from build123d import *

# Parameters (mm, degrees)
F1_DEPTH = 8.45


with BuildPart() as f1:
    # F0 (on Top) → F1 (new body)
    with BuildSketch(Plane.XY):
        with BuildLine():
            Line((-4.005518, -15.555335), (-0.872783, -3.389432))
            ThreePointArc((-0.872783, -3.389432), (-1.979533, -2.886425), (-2.84746, -2.035183))
            Line((-2.84746, -2.035183), (-6.184439, -14.99426))
            ThreePointArc((-6.184439, -14.99426), (-9.390213, -16.435202), (-10.090302, -12.990905))
            Line((-10.090302, -12.990905), (-6.736962, -8.975718))
            Line((-6.736962, -8.975718), (-8.065379, -7.056256))
            Line((-8.065379, -7.056256), (-9.855412, -9.199588))
            Line((-9.855412, -9.199588), (-9.921916, -9.279217))
            Line((-9.921916, -9.279217), (-11.817244, -11.548626))
            ThreePointArc((-11.817244, -11.548626), (-10.417067, -18.437219), (-4.005518, -15.555335))
        make_face()
        Polygon((-9.855412, -9.199588), (-8.065379, -7.056256), (-8.081104, -7.033535), (-9.929378, -4.36292), (-12.83781, -7.845389), align=None)
    extrude(amount=F1_DEPTH)


solid = f1.part
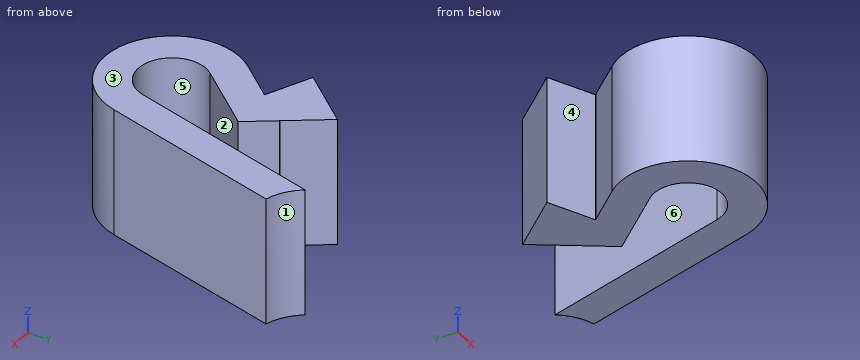
Geometry check sheet. Reference: the model listing, model coordinates, mm. Face numbers are marked on the shaded views. A direction names the side the tool comes from. Give positions to 0.01 mm unless a question says otherwise; leave off trailing zeros. Order: outer loops, then holes, each group sorted by start corner. A loop starts at its lowest first (then second) coordinate and runs counter-clockwise, first axis right, second up. Notation, with made-up numbers: (-39, 16.5) - (-7, 16.5) arc R35 ccw to (-7, 49.5) - close; hole circle Ø5 at (-0.5, 65.25). An arc over 180 degrees is marked (long way). Use one line per item in the form item = value.
1) Sectioned sample at A-A (x = -11). Record the boundary of the cut face in (y, z).
Working result:
outline = (-18.08, 0) - (-10.57, 0) - (-10.57, 8.45) - (-18.08, 8.45) - close; (-8.68, 0) - (-5.64, 0) - (-5.64, 8.45) - (-8.68, 8.45) - close
2) Sectioned sample at B-B (y = -10). Record the boundary of the cut face in (x, z).
Working result:
outline = (-10.52, 0) - (-7.59, 0) - (-7.59, 8.45) - (-10.52, 8.45) - close; (-4.9, 0) - (-2.58, 0) - (-2.58, 8.45) - (-4.9, 8.45) - close
3) Draft check along X on the marked faces 1, 2, 3 and 4. Enter one of: released by +X, released by -X, zero draft, split by the parting line, or undercut.
Working result:
face_1 = released by +X
face_2 = undercut
face_3 = zero draft
face_4 = released by -X
4) Access from +Z, -Z, +X, -X, +Y, -Y to the whole of each face (thin tool, end or side, straight path). Record for the marked faces 5 and 6.
Working result:
face_5 = +Z, -Z
face_6 = +Z, -Z, +Y
5) Material ranges on probe 1 along Y at (x, z) = (-10, 2.5); probe 2 along X at (y, z) = (-14, 4); probe 3 along X at (y, z) = (-4.5, 2.5), recorded low to high. Write a range as from..to.
Working result:
probe_1 = -18.63..-15.98, -12.88..-9.37, -9.13..-4.45
probe_2 = -12.84..-10.57, -5.93..-3.61
probe_3 = -10.04..-9.83, -3.48..-1.16
6) Sectioned sample at D-D (x = -2.5). Record the boundary of the cut face in (y, z).
Working result:
outline = (-9.71, 0) - (-2.45, 0) - (-2.45, 8.45) - (-9.71, 8.45) - close
7) Depth check by flat-ended pin: pin 1 Ø3 at (y, z) = (-12.5, 5.5) entering from +X; pin 2 Ø5 at (x, z) = (-5, 3) entering from -Y; pin 3 Ø5 at (y, z) = (-7.5, 5.5) entering from +X. Enter the tip coordinate at first touch or a pass-through.
Working result:
pin_1 = -2.83
pin_2 = -18.85
pin_3 = -1.29
